Autodesk Fusion 360 part; units mm, degrees
sketch "Sketch1" plane through (0, 0, 0) normal (0, 1, 0) x (1, 0, 0)
  line L0 (0, -1.2) -> (0, 5)
  line L1 (-2.15, 0) -> (-2.0756, -0.85)
  line L2 (-2.15, 0) -> (-0.8392, 0)
  arc A0 (-2.0756, -0.85) -> (0, -1.2) centre (0, 5.1297) ccw
  line L3 (0, 5) -> (-1, 5)
  line L4 (-1, 5) -> (-1, 0.75)
  line L5 (-1, 0.75) -> (-0.8392, 0.15)
  line L6 (-0.8392, 0.15) -> (-0.8392, 0)
  dimension "d13" = 5
  dimension "d14" = 4.3
  dimension "d18" = 2
  dimension "d23" = 15
  dimension "d53" = 1.2
  dimension "d55" = 4.25
  dimension "d56" = 5
  dimension "d57" = 4.85
  dimension "d60" = 0.85
revolve "Revolve1" add sketch "Sketch1" angle 360 about axis through (0, 0, 1.2) along (0, 0, -1) makes body 1
fillet "Fillet2" radius 0.1 1 edges at (-0.7824, 0.3035, 0) on bodies 1
ref_plane "WorkPlane1" through (0, 0, 1.2) normal (0, 0, 1) x (1, 0, 0)
sketch "Sketch2" plane through (0, 0, 1.2) normal (0, 0, 1) x (1, 0, 0)
  line L0 (-1.1, 0) -> (1.1, 0) construction
  line L1 (0, -1.1) -> (0, 1.1) construction
  line L2 (-0.248, 1.1) -> (0.248, 1.1)
  line L3 (0.248, 1.1) -> (0.248, 0.248)
  line L4 (0.248, 0.248) -> (1.1, 0.248)
  line L5 (1.1, 0.248) -> (1.1, -0.248)
  line L6 (1.1, -0.248) -> (0.248, -0.248)
  line L7 (0.248, -0.248) -> (0.248, -1.1)
  line L8 (0.248, -1.1) -> (-0.248, -1.1)
  line L9 (-0.248, -1.1) -> (-0.248, -0.248)
  line L10 (-0.248, -0.248) -> (-1.1, -0.248)
  line L11 (-1.1, -0.248) -> (-1.1, 0.248)
  line L12 (-1.1, 0.248) -> (-0.248, 0.248)
  line L13 (-0.248, 0.248) -> (-0.248, 1.1)
  dimension "d58" = 0.496
  dimension "d59" = 0.496
  dimension "d61" = 2.2
  dimension "d62" = 2.2
extrude "Extrude1" add sketch "Sketch2" against normal blind 1.01 separate body makes body 2
draft "Draft1" angle -30 neutral plane through (0, 0, 1.2) pull (0, 0, 1) 4 faces at (0.0827, -1.1, 0.8633) (-0.0827, 1.1, 0.8633) (-1.1, -0.0827, 0.8633) (1.1, 0.0827, 0.8633) on bodies 2
fillet "Fillet1" radius 0.496 4 edges at (0.248, -0.248, 0.695) (-0.248, -0.248, 0.695) (-0.248, 0.248, 0.695) (0.248, 0.248, 0.695) on bodies 2
combine "Combine1" operation cut target body 1 tool bodies 2
thread "Thread1" thread offset 0 thread length 10
equation "adsk_nomdia = 2.00 mm"
equation "adsk_nomlen = 5.00 mm"
equation "adsk_headdia = 4.30 mm"
equation "adsk_baseh = 0.85 mm"
equation "adsk_phildia = 2.20 mm"
equation "adsk_midfillet = 0.10 mm"
equation "adsk_thrlen = 4.25 mm"
equation "adsk_phildepth = 1.01 mm"
equation "adsk_thrrun = 0.60 mm"
equation "adsk_thrang = 15.00 deg"
equation "adsk_headang = 5.00 deg"
equation "d13 = adsk_headang"
equation "d14 = adsk_headdia"
equation "adsk_ovalh = 0.35 mm"
equation "d18 = adsk_nomdia"
equation "d23 = adsk_thrang"
equation "d32 = adsk_baseh + adsk_ovalh"
equation "adsk_philwidth = 0.496 mm"
equation "d48 = adsk_philwidth"
equation "d52 = adsk_midfillet"
equation "d53 = adsk_baseh + adsk_ovalh"
equation "d55 = adsk_thrlen"
equation "d56 = adsk_nomlen"
equation "d57 = adsk_thrlen + adsk_thrrun"
equation "d58 = adsk_philwidth"
equation "d59 = adsk_philwidth"
equation "d60 = adsk_baseh"
equation "d61 = adsk_phildia"
equation "d62 = adsk_phildia"
properties part number "arrangementsContainer"
The model under review builds one solid part; all positions refer to its coordinate system, in mm. A direction names the side the tool comes from. Round coordinates to 2 decimals unless told otherwise and drop trailing zeros. Write each loop counter-clockwise with the first axis right and the second up, starting at its lowest first coordinate (ties: lowest second). Pieces come first, ordered by that corner, then holes. Notation, with made-up numbers: M 2.25,-32.75 L 33.25,-32.75 A17 cw 33.25,-18.75 Z; hole C -9.75,47.5 d6. An arc over 180 degrees is marked long. Use CSV: the item, a comma, the result in double quotes. Start each with the question number.
(1) For line 1 along Z through (x, y) = (0.3, 1.55); line 2 along Z through (x, y) = (0.3, -0.15); line 3 along X through (y, z) = (-0.9, -1.5), list the stretches that pass through material, from the lowest coordinate up.
(2) We need section A-A, the plane z = 0.5. State the section outline as (x, y) points, then the cut area to 3 significant figures.
(3) We need section B-B, the plane z = -4.5. State the section outline as (x, y) points.
(4) The part is to be moulded in two halves that separate along Y. For faces 3 (the face through (0, 0, 0.19)), 4 (the face through (0.455, -2.047, 0.608)), 5 (the face through (1, -1, 0)), say which applies: +Y half, -Y half, draft (parallel to the pull), parting line (faces both ways), or undercut.
(5) Clearance check with flat-ended pins moving along their axes: P1, Ø1, axis at y = -1, z = -3.5, coming from the +X side; P2, Ø0.5, axis at x = 0, y = 0, coming from the +Z side. State where each tip first meets the part, or that it passes through.
(6) Tool access review of faces 1 (the face through (0, 1, -3)), 2 (the face through (0, 0, -5)): name each direction out of +Z, -Z, +X, -X, +Y, -Y from which nothing blocks a thin tool from reaching the whole face with its end or side.
(7) We need section C-C, the plane z = -0.5. State the section outline as (x, y) points, then the cut area to 3 significant figures.
Findings:
1,line 1,"0 to 1"
1,line 2,"-5 to 0.19"
1,line 3,"-0.44 to 0.44"
2,outline,"C 0,0 d4.21; hole M -0.7,-0.25 A0.5 cw -0.25,-0.7 L 0.25,-0.7 A0.5 cw 0.7,-0.25 L 0.7,0.25 A0.5 cw 0.25,0.7 L -0.25,0.7 A0.5 cw -0.7,0.25 Z"
2,area,"12.6 mm^2"
3,outline,"C 0,0 d2"
4,face 3,"undercut"
4,face 4,"parting line"
4,face 5,"draft"
5,P1,"x = 0.87"
5,P2,"z = 0.19"
6,face 1,"-Z"
6,face 2,"-Z, +X, -X, +Y, -Y"
7,outline,"C 0,0 d1.87"
7,area,"2.73 mm^2"
